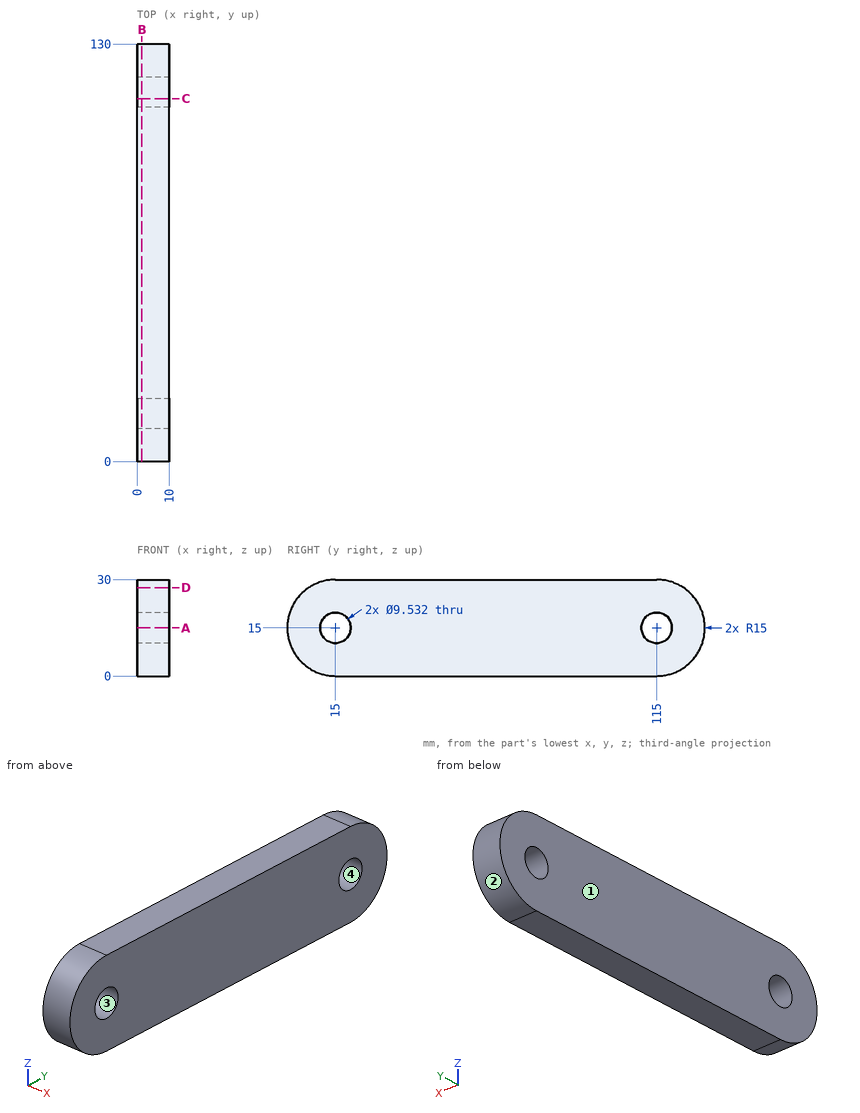
Geometry: see drawing. Coordinates: mm, zero at the bounding-box minimum. Round coordinates to 2 decimals unless told otherwise and drop trailing zeros. Order: outer loops, then holes, each group sorted by start corner. A loop starts at its lowest first (then second) coordinate and runs counter-clockwise, first axis right, second up. Notation, with made-up numbers: (-7.75, 62.25) -> (11.25, 62.25) arc R11 ccw to (11.25, 66.25) -> close; hole circle Ø11 at (61.5, 37). An arc over 180 degrees is marked (long way). Answer as CSV lines item,"result".
Item 1: Section B-B, the plane x = 1.5. Return loops of the section in (y, z), plus the area to 3 significant figures.
A:
outline,"(15, 0) -> (115, 0) arc R15 ccw to (115, 30) -> (15, 30) arc R15 ccw to start; hole circle Ø9.53 at (15, 15); hole circle Ø9.53 at (115, 15)"
area,"3,560 mm²"
Item 2: Line query: L1, parallel to Y at x = 6.25, z = 15; L2, parallel to Z at x = 8, y = 15; L3, parallel to Y at x = 4, z = 17. Output: solid intervals per line, ascending.
A:
L1,"0 to 10.23, 19.77 to 110.23, 119.77 to 130"
L2,"0 to 10.23, 19.77 to 30"
L3,"0.13 to 10.67, 19.33 to 110.67, 119.33 to 129.87"
Item 3: Section C-C, the plane y = 113. Return loops of the section in (x, z).
A:
outline,"(0, 0) -> (10, 0) -> (10, 10.67) -> (0, 10.67) -> close; (0, 19.33) -> (10, 19.33) -> (10, 30) -> (0, 30) -> close"
Item 4: Section D-D, the plane z = 27.5. Return loops of the section in (x, y), plus the area to 3 significant figures.
A:
outline,"(0, 6.71) -> (10, 6.71) -> (10, 123.29) -> (0, 123.29) -> close"
area,"1,170 mm²"
Item 5: Pin query (flat end, axial travel): pin 1 Ø3 at (x, z) = (1.5, 10.5) entering from -Y; pin 2 Ø2 at (x, z) = (6.5, 12) entering from -Y; pin 3 Ø8.5 at (y, z) = (115, 15) entering from -X. Return the tip coordinate at first contact, or that it passes through.
A:
pin 1,"y = 0.3"
pin 2,"y = 0.13"
pin 3,"through"
Item 6: Pull-direction query (Y, two-part tool) for the marked faces 1, 2, 3 and 4; classes: pulls with the +Y half, pulls with the -Y half, needs draft (parallel to the pull), parting line crosses it, or undercut.
A:
face 1,"needs draft"
face 2,"pulls with the +Y half"
face 3,"undercut"
face 4,"undercut"
Item 7: Section A-A, the plane z = 15. Return loops of the section in (x, y), plus the area to 3 significant figures.
A:
outline,"(0, 0) -> (10, 0) -> (10, 10.23) -> (0, 10.23) -> close; (0, 19.77) -> (10, 19.77) -> (10, 110.23) -> (0, 110.23) -> close; (0, 119.77) -> (10, 119.77) -> (10, 130) -> (0, 130) -> close"
area,"1,110 mm²"
